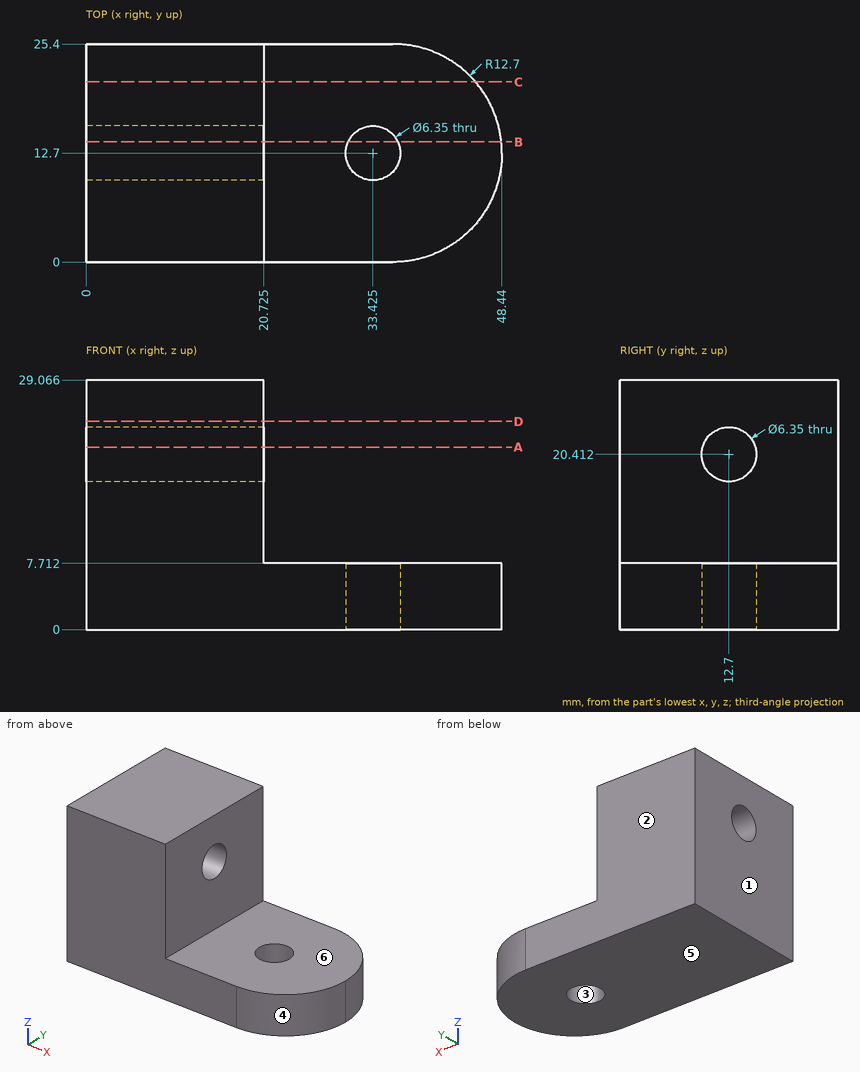
The figure shows three views and two pictorial views of one solid part (mm, origin at its lowest corner). Answer the questions. A direction names the side the tool comes from. Coordinates: 2 decimals unless noted, no trailing zeros. Order: outer loops, then holes, each group sorted by start corner. A loop starts at its lowest first (then second) coordinate and runs counter-clockwise, first axis right, second up.
Q1. For a pull along X with two mould halves and no side action, classify the marked faces 1, 2, 3 and 4 as pulls with the +X half, pulls with the -X half, needs draft (parallel to the pull), parting line crosses it, or undercut.
Q2. A cutting plane is placed at C-C, the plane y = 21. Write down the section's boundary in (x, z) (1 decimal), and give its area (3 significant figures).
Q3. A cutting plane is placed at A-A, the plane z = 21.25. Write down the section's boundary in (x, y) (1 decimal).
Q4. A cutting plane is placed at D-D, the plane z = 24.25. Write down the section's boundary in (x, y) (1 decimal).
Q5. Which of the six approach directions +Z, -Z, +X, -X, +Y, -Y give full straight-line access (tool end or side, diameter ignored) to the marked faces 5 and 6?
Q6. Given P1, Ø10.5, axis at y = 13.5, z = 17, coming from the +X side (1 decimal); P2, Ø3, axis at x = 27.5, y = 17, coming from the +Z side; P3, Ø6, axis at x = 42.5, z = 6.5, coming from the +Y side; P4, Ø5.5, axis at x = 33.43, y = 12.7, coming from the +Z side, each flat-ended and moving along its own axis, determine where each tip first touches the part or whether it passes through.
Q7. Consider line 1 (Z direction, x = 9.5, y = 12.7) (1 decimal); line 2 (Z direction, x = 21, y = 16); line 3 (X direction, y = 17.5, z = 19.75) (1 decimal). Determine where each line is inside the solid, lowest interval first.
Q8. A cutting plane is placed at B-B, the plane y = 14. Write down the section's boundary in (x, z) (1 decimal).
Answers follow:
1. face 1: pulls with the -X half
1. face 2: needs draft
1. face 3: undercut
1. face 4: pulls with the +X half
2. outline: (0, 0) - (45.4, 0) - (45.4, 7.7) - (20.7, 7.7) - (20.7, 29.1) - (0, 29.1) - close
2. area: 792 mm2
3. outline: (0, 0) - (20.7, 0) - (20.7, 9.6) - (0, 9.6) - close; (0, 15.8) - (20.7, 15.8) - (20.7, 25.4) - (0, 25.4) - close
4. outline: (0, 0) - (20.7, 0) - (20.7, 25.4) - (0, 25.4) - close
5. face 5: -Z, +X, -X, +Y, -Y
5. face 6: +Z, +X, +Y, -Y
6. P1: stops at x = 20.7
6. P2: stops at z = 7.71
6. P3: stops at y = 24.83
6. P4: passes through
7. line 1: z = 0 to 17.2, 23.6 to 29.1
7. line 2: z = 0 to 7.71
7. line 3: x = 0 to 20.7
8. outline: (0, 0) - (30.5, 0) - (30.5, 7.7) - (20.7, 7.7) - (20.7, 17.5) - (0, 17.5) - close; (0, 23.3) - (20.7, 23.3) - (20.7, 29.1) - (0, 29.1) - close; (36.3, 0) - (48.4, 0) - (48.4, 7.7) - (36.3, 7.7) - close
